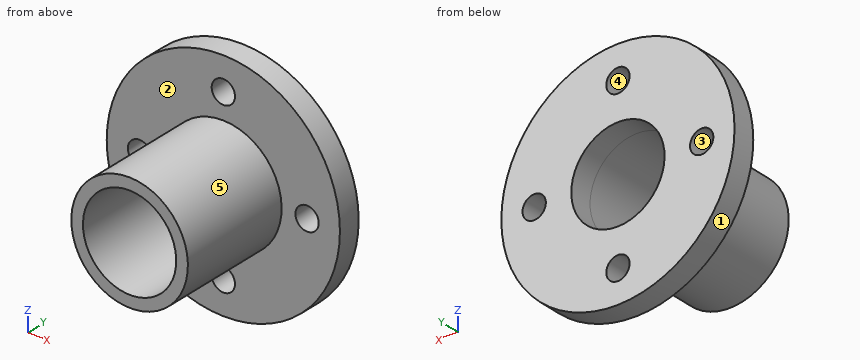
from build123d import *

# Parameters (mm, degrees)
SKETCH1_R           = 5
SKETCH1_R_2         = 4
BOSS_EXTRUDE1_DEPTH = 10
SKETCH2_R           = 10
BOSS_EXTRUDE2_DEPTH = 2
SKETCH3_R           = 1
CUT_EXTRUDE1_DEPTH  = 2
SKETCH4_R           = 4
CUT_EXTRUDE2_DEPTH  = 2


with BuildPart() as part:
    # Sketch1 → Boss-Extrude1 (new body)
    with BuildSketch(Plane(origin=(0, 0, 0), x_dir=(1, 0, 0), z_dir=(0, 1, 0))):
        with Locations(Location((0, 0, 0), (0, 0, 270))):
            Circle(SKETCH1_R)
        with Locations(Location((0, 0, 0), (0, 0, 270))):
            Circle(SKETCH1_R_2, mode=Mode.SUBTRACT)
    extrude(amount=BOSS_EXTRUDE1_DEPTH)

    # Sketch2 → Boss-Extrude2 (add)
    with BuildSketch(Plane(origin=(0, 10, 0), x_dir=(1, 0, 0), z_dir=(0, 1, 0))):
        with Locations(Location((0, 0, 0), (0, 0, 270))):
            Circle(SKETCH2_R)
    extrude(amount=BOSS_EXTRUDE2_DEPTH)

    # Sketch3 → Cut-Extrude1 (cut)
    with BuildSketch(Plane(origin=(0, 10, 0), x_dir=(-1, 0, 0), z_dir=(0, -1, 0))):
        with Locations(Location((-7.183252609, 0, 0), (0, 0, 90))):
            Circle(SKETCH3_R)
        with Locations(Location((0, 7.183252609, 0), (0, 0, 90))):
            Circle(SKETCH3_R)
        with Locations(Location((7.183252609, 0, 0), (0, 0, 90))):
            Circle(SKETCH3_R)
        with Locations(Location((0, -7.183252609, 0), (0, 0, 90))):
            Circle(SKETCH3_R)
    extrude(amount=-CUT_EXTRUDE1_DEPTH, mode=Mode.SUBTRACT)

    # Sketch4 → Cut-Extrude2 (cut)
    with BuildSketch(Plane(origin=(0, 10, 0), x_dir=(-1, 0, 0), z_dir=(0, -1, 0))):
        with Locations(Location((0, 0, 0), (0, 0, 90))):
            Circle(SKETCH4_R)
    extrude(amount=-CUT_EXTRUDE2_DEPTH, mode=Mode.SUBTRACT)


solid = part.part
Design review of the part built by this model. Coordinates are the model's own, in mm. Face numbers are marked on the shaded views. A direction names the side the tool comes from. Coordinates: 2 decimals unless noted, no trailing zeros. Write each loop counter-clockwise with the first axis right and the second up, starting at its lowest first coordinate (ties: lowest second). Pieces come first, ordered by that corner, then holes. Notation, with made-up numbers: (49, 41) - (72, 41) arc R28 ccw to (72, 76) - close; hole circle Ø4 at (-9, 89). An arc over 180 degrees is marked (long way). Use one line per item in the form item = value.
Q1. Consider section D-D (y = 3.5). Write out the cut boundary in (x, z).
Taken from the geometry:
outline = circle Ø10 at (0, 0); hole circle Ø8 at (0, 0)
Q2. Machinability: for the marked faces 4 and 5, which of the approach directions +Z, -Z, +X, -X, +Y, -Y give a long, thin tool a straight path to every point of the face, cutting with its end or side? Answer none if there is none.
Taken from the geometry:
face_4 = +Y, -Y
face_5 = -Y
Q3. The part is to be moulded in two halves that separate along Z. For the marked faces 1, 2 and 3, say which applies: +Z half, -Z half, draft (parallel to the pull), parting line (faces both ways), or undercut.
Taken from the geometry:
face_1 = parting line
face_2 = draft
face_3 = undercut
Q4. Consider section C-C (z = -3). Write out the cut boundary in (x, y).
Taken from the geometry:
outline = (-9.54, 10) - (-4, 10) - (-4, 0) - (-2.65, 0) - (-2.65, 12) - (-9.54, 12) - close; (2.65, 0) - (4, 0) - (4, 10) - (9.54, 10) - (9.54, 12) - (2.65, 12) - close
Q5. Consider section B-B (z = 0). Write out the cut boundary in (x, y), plus the area to 3 significant figures.
Taken from the geometry:
outline = (-10, 10) - (-8.18, 10) - (-8.18, 12) - (-10, 12) - close; (-6.18, 10) - (-5, 10) - (-5, 0) - (-4, 0) - (-4, 12) - (-6.18, 12) - close; (4, 0) - (5, 0) - (5, 10) - (6.18, 10) - (6.18, 12) - (4, 12) - close; (8.18, 10) - (10, 10) - (10, 12) - (8.18, 12) - close
area = 36.0 mm^2
Q6. Consider section A-A (x = 0). Write out the cut boundary in (y, z).
Taken from the geometry:
outline = (0, -5) - (10, -5) - (10, -6.18) - (12, -6.18) - (12, -4) - (0, -4) - close; (0, 4) - (12, 4) - (12, 6.18) - (10, 6.18) - (10, 5) - (0, 5) - close; (10, -10) - (12, -10) - (12, -8.18) - (10, -8.18) - close; (10, 8.18) - (12, 8.18) - (12, 10) - (10, 10) - close
Q7. For probe 1 along X at (y, z) = (10.7, 0); probe 2 along Y at (x, z) = (-8, 3.75); probe 3 along X at (y, z) = (3.5, 0), list the stretches that pass through material, from the lowest coordinate up.
Taken from the geometry:
probe_1 = -10 to -8.18, -6.18 to -4, 4 to 6.18, 8.18 to 10
probe_2 = 10 to 12
probe_3 = -5 to -4, 4 to 5
Q8. Insertion check: pin 1 Ø1.2 at (x, z) = (0, -7.18) entering from +Y. The pin has a flat end and moves straight along its axis. Give the tip position at first contact, or say it passes through.
Taken from the geometry:
pin_1 = through
